Autodesk Inventor part; units mm, degrees
ref_plane "YZ Plane" through (0, 0, 0) normal (1, 0, 0) x (0, 1, 0)
ref_plane "XZ Plane" through (0, 0, 0) normal (0, 1, 0) x (-1, 0, 0)
ref_plane "XY Plane" through (0, 0, 0) normal (0, 0, 1) x (1, 0, 0)
sketch "Sketch1" plane through (0, 0, 0) normal (0, 0, 1) x (1, 0, 0)
  circle A0 centre (0, 0) radius 17.25
  circle A1 centre (0, 0) radius 16.1
  circle A2 centre (0, 0) radius 15
  line L0 (-1.25, -15.0046) -> (1.25, -15.0046)
  line L1 (-1.75, -16.0046) -> (1.75, -16.0046)
  line L2 (1.75, -16.0046) -> (1.25, -15.0046)
  line L3 (-1.75, -16.0046) -> (-1.25, -15.0046)
  line L4 (-1.25, -15.0046) -> (-1.2227, -14.9501)
  line L5 (1.25, -15.0046) -> (1.2227, -14.9501)
  line L6 (2.6761, -14.8169) -> (5.0909, -14.1698)
  line L7 (2.4519, -15.9122) -> (2.6761, -14.8169)
  line L8 (2.6761, -14.8169) -> (2.6883, -14.7571)
  line L9 (5.8327, -15.0063) -> (5.0909, -14.1698)
  line L10 (5.0909, -14.1698) -> (5.0504, -14.1242)
  line L11 (6.4198, -13.6194) -> (8.5848, -12.3694)
  line L12 (6.4868, -14.7354) -> (6.4198, -13.6194)
  line L13 (6.4198, -13.6194) -> (6.4161, -13.5585)
  line L14 (9.5178, -12.9854) -> (8.5848, -12.3694)
  line L15 (8.5848, -12.3694) -> (8.534, -12.3358)
  line L16 (9.726, -11.4937) -> (11.4937, -9.726)
  line L17 (10.0795, -12.5544) -> (9.726, -11.4937)
  line L18 (9.726, -11.4937) -> (9.7067, -11.4359)
  line L19 (12.5544, -10.0795) -> (11.4937, -9.726)
  line L20 (11.4937, -9.726) -> (11.4359, -9.7067)
  line L21 (12.3694, -8.5848) -> (13.6194, -6.4198)
  line L22 (12.9854, -9.5178) -> (12.3694, -8.5848)
  line L23 (12.3694, -8.5848) -> (12.3358, -8.534)
  line L24 (14.7354, -6.4868) -> (13.6194, -6.4198)
  line L25 (13.6194, -6.4198) -> (13.5585, -6.4161)
  line L26 (14.1698, -5.0909) -> (14.8169, -2.6761)
  line L27 (15.0063, -5.8327) -> (14.1698, -5.0909)
  line L28 (14.1698, -5.0909) -> (14.1242, -5.0504)
  line L29 (15.9122, -2.4519) -> (14.8169, -2.6761)
  line L30 (14.8169, -2.6761) -> (14.7571, -2.6883)
  line L31 (15.0046, -1.25) -> (15.0046, 1.25)
  line L32 (16.0046, -1.75) -> (15.0046, -1.25)
  line L33 (15.0046, -1.25) -> (14.9501, -1.2227)
  line L34 (16.0046, 1.75) -> (15.0046, 1.25)
  line L35 (15.0046, 1.25) -> (14.9501, 1.2227)
  line L36 (14.8169, 2.6761) -> (14.1698, 5.0909)
  line L37 (15.9122, 2.4519) -> (14.8169, 2.6761)
  line L38 (14.8169, 2.6761) -> (14.7571, 2.6883)
  line L39 (15.0063, 5.8327) -> (14.1698, 5.0909)
  line L40 (14.1698, 5.0909) -> (14.1242, 5.0504)
  line L41 (13.6194, 6.4198) -> (12.3694, 8.5848)
  line L42 (14.7354, 6.4868) -> (13.6194, 6.4198)
  line L43 (13.6194, 6.4198) -> (13.5585, 6.4161)
  line L44 (12.9854, 9.5178) -> (12.3694, 8.5848)
  line L45 (12.3694, 8.5848) -> (12.3358, 8.534)
  line L46 (11.4937, 9.726) -> (9.726, 11.4937)
  line L47 (12.5544, 10.0795) -> (11.4937, 9.726)
  line L48 (11.4937, 9.726) -> (11.4359, 9.7067)
  line L49 (10.0795, 12.5544) -> (9.726, 11.4937)
  line L50 (9.726, 11.4937) -> (9.7067, 11.4359)
  line L51 (8.5848, 12.3694) -> (6.4198, 13.6194)
  line L52 (9.5178, 12.9854) -> (8.5848, 12.3694)
  line L53 (8.5848, 12.3694) -> (8.534, 12.3358)
  line L54 (6.4868, 14.7354) -> (6.4198, 13.6194)
  line L55 (6.4198, 13.6194) -> (6.4161, 13.5585)
  line L56 (5.0909, 14.1698) -> (2.6761, 14.8169)
  line L57 (5.8327, 15.0063) -> (5.0909, 14.1698)
  line L58 (5.0909, 14.1698) -> (5.0504, 14.1242)
  line L59 (2.4519, 15.9122) -> (2.6761, 14.8169)
  line L60 (2.6761, 14.8169) -> (2.6883, 14.7571)
  line L61 (1.25, 15.0046) -> (-1.25, 15.0046)
  line L62 (1.75, 16.0046) -> (1.25, 15.0046)
  line L63 (1.25, 15.0046) -> (1.2227, 14.9501)
  line L64 (-1.75, 16.0046) -> (-1.25, 15.0046)
  line L65 (-1.25, 15.0046) -> (-1.2227, 14.9501)
  line L66 (-2.6761, 14.8169) -> (-5.0909, 14.1698)
  line L67 (-2.4519, 15.9122) -> (-2.6761, 14.8169)
  line L68 (-2.6761, 14.8169) -> (-2.6883, 14.7571)
  line L69 (-5.8327, 15.0063) -> (-5.0909, 14.1698)
  line L70 (-5.0909, 14.1698) -> (-5.0504, 14.1242)
  line L71 (-6.4198, 13.6194) -> (-8.5848, 12.3694)
  line L72 (-6.4868, 14.7354) -> (-6.4198, 13.6194)
  line L73 (-6.4198, 13.6194) -> (-6.4161, 13.5585)
  line L74 (-9.5178, 12.9854) -> (-8.5848, 12.3694)
  line L75 (-8.5848, 12.3694) -> (-8.534, 12.3358)
  line L76 (-9.726, 11.4937) -> (-11.4937, 9.726)
  line L77 (-10.0795, 12.5544) -> (-9.726, 11.4937)
  line L78 (-9.726, 11.4937) -> (-9.7067, 11.4359)
  line L79 (-12.5544, 10.0795) -> (-11.4937, 9.726)
  line L80 (-11.4937, 9.726) -> (-11.4359, 9.7067)
  line L81 (-12.3694, 8.5848) -> (-13.6194, 6.4198)
  line L82 (-12.9854, 9.5178) -> (-12.3694, 8.5848)
  line L83 (-12.3694, 8.5848) -> (-12.3358, 8.534)
  line L84 (-14.7354, 6.4868) -> (-13.6194, 6.4198)
  line L85 (-13.6194, 6.4198) -> (-13.5585, 6.4161)
  line L86 (-14.1698, 5.0909) -> (-14.8169, 2.6761)
  line L87 (-15.0063, 5.8327) -> (-14.1698, 5.0909)
  line L88 (-14.1698, 5.0909) -> (-14.1242, 5.0504)
  line L89 (-15.9122, 2.4519) -> (-14.8169, 2.6761)
  line L90 (-14.8169, 2.6761) -> (-14.7571, 2.6883)
  line L91 (-15.0046, 1.25) -> (-15.0046, -1.25)
  line L92 (-16.0046, 1.75) -> (-15.0046, 1.25)
  line L93 (-15.0046, 1.25) -> (-14.9501, 1.2227)
  line L94 (-16.0046, -1.75) -> (-15.0046, -1.25)
  line L95 (-15.0046, -1.25) -> (-14.9501, -1.2227)
  line L96 (-14.8169, -2.6761) -> (-14.1698, -5.0909)
  line L97 (-15.9122, -2.4519) -> (-14.8169, -2.6761)
  line L98 (-14.8169, -2.6761) -> (-14.7571, -2.6883)
  line L99 (-15.0063, -5.8327) -> (-14.1698, -5.0909)
  line L100 (-14.1698, -5.0909) -> (-14.1242, -5.0504)
  line L101 (-13.6194, -6.4198) -> (-12.3694, -8.5848)
  line L102 (-14.7354, -6.4868) -> (-13.6194, -6.4198)
  line L103 (-13.6194, -6.4198) -> (-13.5585, -6.4161)
  line L104 (-12.9854, -9.5178) -> (-12.3694, -8.5848)
  line L105 (-12.3694, -8.5848) -> (-12.3358, -8.534)
  line L106 (-11.4937, -9.726) -> (-9.726, -11.4937)
  line L107 (-12.5544, -10.0795) -> (-11.4937, -9.726)
  line L108 (-11.4937, -9.726) -> (-11.4359, -9.7067)
  line L109 (-10.0795, -12.5544) -> (-9.726, -11.4937)
  line L110 (-9.726, -11.4937) -> (-9.7067, -11.4359)
  line L111 (-8.5848, -12.3694) -> (-6.4198, -13.6194)
  line L112 (-9.5178, -12.9854) -> (-8.5848, -12.3694)
  line L113 (-8.5848, -12.3694) -> (-8.534, -12.3358)
  line L114 (-6.4868, -14.7354) -> (-6.4198, -13.6194)
  line L115 (-6.4198, -13.6194) -> (-6.4161, -13.5585)
  line L116 (-5.0909, -14.1698) -> (-2.6761, -14.8169)
  line L117 (-5.8327, -15.0063) -> (-5.0909, -14.1698)
  line L118 (-5.0909, -14.1698) -> (-5.0504, -14.1242)
  line L119 (-2.4519, -15.9122) -> (-2.6761, -14.8169)
  line L120 (-2.6761, -14.8169) -> (-2.6883, -14.7571)
  point P0 (0, -16.0046)
  point P1 (0, -15.0046)
  point P2 (1.75, -16.0046)
  point P3 (3.8835, -14.4933)
  point P4 (7.5023, -12.9944)
  point P5 (10.6099, -10.6099)
  point P6 (12.9944, -7.5023)
  point P7 (14.4933, -3.8835)
  point P8 (15.0046, 0)
  point P9 (14.4933, 3.8835)
  point P10 (12.9944, 7.5023)
  point P11 (10.6099, 10.6099)
  point P12 (7.5023, 12.9944)
  point P13 (3.8835, 14.4933)
  point P14 (0, 15.0046)
  point P15 (-3.8835, 14.4933)
  point P16 (-7.5023, 12.9944)
  point P17 (-10.6099, 10.6099)
  point P18 (-12.9944, 7.5023)
  point P19 (-14.4933, 3.8835)
  point P20 (-15.0046, 0)
  point P21 (-14.4933, -3.8835)
  point P22 (-12.9944, -7.5023)
  point P23 (-10.6099, -10.6099)
  point P24 (-7.5023, -12.9944)
  point P25 (-3.8835, -14.4933)
  dimension "d1" = 32.2
  dimension "d0" = 34.5
  dimension "d2" = 30
  dimension "d3" = 2.5
  dimension "d4" = 3.5
  dimension "d5" = 1
  dimension "d20" = 360
extrude "Extrusion1" add sketch "Sketch1" along normal blind 15 contours L34 L35 A2 L38 L37 A1 | A1 L29 L30 A2 L33 L32 | L31 L33 A2 L35 | L39 L40 A2 L43 L42 A1 | L38 A2 L40 L36 | A2 | A1 L24 L25 A2 L28 L27 | L26 L28 A2 L30 | L44 L45 A2 L48 L47 A1 | L43 A2 L45 L41 | A1 L19 L20 A2 L23 L22 | L21 L23 A2 L25 | L49 L50 A2 L53 L52 A1 | L48 A2 L50 L46 | A1 L14 L15 A2 L18 L17 | L16 L18 A2 L20 | L54 L55 A2 L58 L57 A1 | L53 A2 L55 L51 | A1 L9 L10 A2 L13 L12 | L11 L13 A2 L15 | L59 L60 A2 L63 L62 A1 | L58 A2 L60 L56 | A1 L2 L5 A2 L8 L7 | L6 L8 A2 L10 | L64 L65 A2 L68 L67 A1 | L63 A2 L65 L61 | A1 L119 L120 A2 L4 L3 | L69 L70 A2 L73 L72 A1 | L68 A2 L70 L66 | A1 L114 L115 A2 L118 L117 | L116 L118 A2 L120 | L74 L75 A2 L78 L77 A1 | L73 A2 L75 L71 | A1 L109 L110 A2 L113 L112 | L111 L113 A2 L115 | L79 L80 A2 L83 L82 A1 | L78 A2 L80 L76 | A1 L104 L105 A2 L108 L107 | L106 L108 A2 L110 | L84 L85 A2 L88 L87 A1 | L83 A2 L85 L81 | A1 L99 L100 A2 L103 L102 | L101 L103 A2 L105 | L89 L90 A2 L93 L92 A1 | L88 A2 L90 L86 | A1 L94 L95 A2 L98 L97 | L96 L98 A2 L100 | L93 A2 L95 L91
sketch "Sketch2" plane through (0, 0, 0) normal (0, 0, -1) x (-1, 0, 0)
  line L0 (12, 6.9282) -> (12, -6.9282)
  line L1 (12, -6.9282) -> (0, -13.8564)
  line L2 (0, -13.8564) -> (-12, -6.9282)
  line L3 (-12, -6.9282) -> (-12, 6.9282)
  line L4 (-12, 6.9282) -> (0, 13.8564)
  line L5 (0, 13.8564) -> (12, 6.9282)
  point P0 (0, 0)
  point P1 (0, 0)
  dimension "d12" = 24
extrude "Extrusion2" add sketch "Sketch2" along normal blind 10
sketch "Sketch3" plane through (0, 0, -10) normal (0, 0, -1) x (-1, 0, 0)
  circle A0 centre (0, 0) radius 7.5
  dimension "d15" = 15
extrude "Extrusion3" [suppressed]
sketch "Sketch4" plane through (0, 0, 0) normal (1, 0, 0) x (0, 1, 0)
  line L0 (20.8545, -11.8216) -> (-20.3089, -11.8216)
  line L1 (-20.3089, -11.8216) -> (-20.3089, 5.7592)
  line L2 (-20.3089, 5.7592) -> (20.8545, 5.7592)
  line L3 (20.8545, 5.7592) -> (20.8545, -11.8216)
  point P0 (0, 0)
extrude "Extrusion4" [suppressed]
properties part number "Nastavek Millard freewheel tool vecji trapze"
The listing builds one solid part. Answer for the finished solid, in the listing's coordinates (mm). A direction names the side the tool comes from. Round coordinates to 2 decimals unless told otherwise and drop trailing zeros. Write each loop counter-clockwise with the first axis right and the second up, starting at its lowest first coordinate (ties: lowest second). Pieces come first, ordered by that corner, then holes. Notation, with made-up numbers: M -7.75,57 L 35.25,57 A25 ccw 35.25,75 Z; hole C 20,-1.75 d5. An arc over 180 degrees is marked long. Write each question's results on one line, items separated by ' | '. Start each with the question number.
(1) Determine the mould class of faces 4 (the flat face through (1.503, 15.512, 7.395)), 5 (the flat face through (0, 0, 15)), 6 (the flat face through (-14.49, 3.9, 7.4)) for opening direction Y: +Y half, -Y half, draft (parallel to the pull), parting line (faces both ways), or undercut.
(2) The part is cut by section C-C, the plane y = -7.5. Write down the section's boundary in (x, z), and give its area (3 significant figures).
(3) The part is cut by section B-B, the plane x = -9. Write down the section's boundary in (y, z).
(4) Each of these flat-tipped pins is pushed along its axis until it touches: P1, Ø11, axis at y = 3, z = -7.5, coming from the -X side; P2, Ø1.5, axis at y = 6.5, z = 3.5, coming from the -X side; P3, Ø0.8, axis at y = 0, z = 9.5, coming from the +X side. Where does it stop, or does it pass through?
(5) The part is cut by section A-A, the plane z = -5.5. Write down the section's boundary in (x, y), and give its area (3 significant figures).
(6) Find the intervals of material crossed by line 1 (Z direction, x = -13, y = -4.5); line 2 (Y direction, x = 3, z = 10.25); line 3 (Y direction, x = 11.5, z = 0.75), in increasing order.
(7) For faces 1 (the flat face through (5.92, -10.44, -4.93)), 2 (the flat face through (-14.185, -6.454, 7.395)), 3 (the flat face through (12.682, 9.058, 7.395)), determine the directions among +Z, -Z, +X, -X, +Y, -Y from which every point of the face is accessible in a straight line to the end or side of a thin tool.
Worked answers:
1) face 4: +Y half | face 5: draft | face 6: undercut
2) outline: M -13,0 L -11.01,0 L -11.01,-10 L 11.01,-10 L 11.01,0 L 13,0 L 13,15 L -13,15 Z | area: 610 mm²
3) outline: M -12.64,0 L -8.66,0 L -8.66,-10 L 8.66,-10 L 8.66,0 L 12.64,0 L 12.64,15 L -12.64,15 Z
4) P1: stops at x = -12 | P2: stops at x = -15.01 | P3: stops at x = 15
5) outline: M -12,-6.93 L 0,-13.86 L 12,-6.93 L 12,6.93 L 0,13.86 L -12,6.93 Z | area: 499 mm²
6) line 1: z = 0 to 15 | line 2: y = -14.73 to 14.73 | line 3: y = -9.73 to 9.73
7) face 1: -Z, +X, -Y | face 2: +Z, -Z, -Y | face 3: +Z, -Z, +X
